Geometry check sheet. Reference: the model listing, model coordinates, mm. Face numbers are marked on the shaded views. A direction names the side the tool comes from. Round coordinates to 2 decimals unless told otherwise and drop trailing zeros. Loops run counter-clockwise (first coordinate to the right, second up) from the corner with the lowest first, then second, coordinate; pieces in that order, holes last.
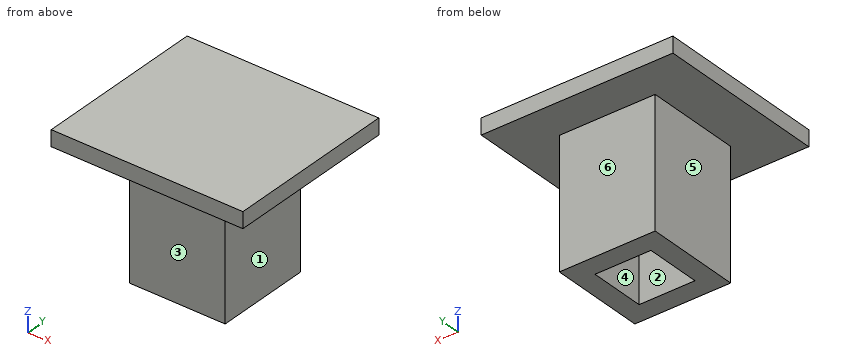
```python
from build123d import *

# Parameters (mm, degrees)
F0_W     = 152.4
F0_H     = 12.7
F1_DEPTH = 137.16
F2_W     = 76.2
F2_H     = 76.2
F3_DEPTH = 101.6
F4_W     = 44.45
F4_H     = 44.45
F5_DEPTH = 101.6


with BuildPart() as f1:
    # F0 (on Front) → F1 (new body)
    with BuildSketch(Plane.XZ):
        with Locations((76.2, 6.35)):
            Rectangle(F0_W, F0_H)
    extrude(amount=F1_DEPTH)

    # F2 (on face) → F3 (join)
    with BuildSketch(Plane(origin=(0, 0, 0), x_dir=(1, 0, 0), z_dir=(0, 0, -1))):
        with Locations((76.2, 68.58)):
            Rectangle(F2_W, F2_H)
    extrude(amount=F3_DEPTH)

    # F4 (on face) → F5 (cut)
    with BuildSketch(Plane(origin=(0, 0, -101.6), x_dir=(1, 0, 0), z_dir=(0, 0, -1))):
        with Locations((76.2, 68.58)):
            Rectangle(F4_W, F4_H)
    extrude(amount=-F5_DEPTH, mode=Mode.SUBTRACT)


solid = f1.part
```
1) Mould release check, pull along X, two halves, no side actions. Record for the marked faces 1, 2 and 3: +X half, -X half, draft (parallel to the pull), parting line (faces both ways), or undercut.
Report:
face 1: +X half
face 2: undercut
face 3: draft
2) Sectioned sample at C-C, the plane x = 50.5. Record the cut outline in (y, z), then the cut area to 3 significant figures.
Report:
outline: (-137.16, 0) - (-106.68, 0) - (-106.68, -101.6) - (-30.48, -101.6) - (-30.48, 0) - (0, 0) - (0, 12.7) - (-137.16, 12.7) - close
area: 9,480 mm2
3) Access from +Z, -Z, +X, -X, +Y, -Y to the whole of each face (thin tool, end or side, straight path). Record for the marked faces 4, 5 and 6.
Report:
face 4: -Z
face 5: -Z, -X, +Y, -Y
face 6: -Z, +X, -X, +Y
4) Sectioned sample at B-B, the plane y = -66.5. Record the cut outline in (x, z) (3 decimals).
Report:
outline: (0, 0) - (38.1, 0) - (38.1, -101.6) - (53.975, -101.6) - (53.975, 0) - (98.425, 0) - (98.425, -101.6) - (114.3, -101.6) - (114.3, 0) - (152.4, 0) - (152.4, 12.7) - (0, 12.7) - close
5) Gauge pin test, flat ends, axial feed: pin 1 (13.5 mm diameter, centred on x = 82, y = -60, fed in from -Z); pin 2 (13.5 mm diameter, centred on x = 72.5, z = -46, fed in from +Y); pin 3 (22 mm diameter, centred on y = -71, z = -70.5, fed in from -X). Record the tip position at first contact, or that the pin passes through.
Report:
pin 1: stops at z = 0
pin 2: stops at y = -30.48
pin 3: stops at x = 38.1
6) Sectioned sample at D-D, the plane y = -42. Record the cut outline in (x, z), then the cut area to 3 significant figures.
Report:
outline: (0, 0) - (38.1, 0) - (38.1, -101.6) - (114.3, -101.6) - (114.3, 0) - (152.4, 0) - (152.4, 12.7) - (0, 12.7) - close
area: 9,680 mm2
7) Sectioned sample at A-A, the plane z = -71. Record the cut outline in (x, y) (3 decimals), then the cut area to 3 significant figures.
Report:
outline: (38.1, -106.68) - (114.3, -106.68) - (114.3, -30.48) - (38.1, -30.48) - close; hole (53.975, -90.805) - (98.425, -90.805) - (98.425, -46.355) - (53.975, -46.355) - close
area: 3,830 mm2
8) Scan lines: line 1 along X through (y, z) = (-83, -47.5) (3 decimals); line 2 along Y through (x, z) = (73, -25) (3 decimals); line 3 along Z through (x, y) = (92, -10.5). Record each from-to range of solid material in increasing order.
Report:
line 1: x = 38.1 to 53.975, 98.425 to 114.3
line 2: y = -106.68 to -90.805, -46.355 to -30.48
line 3: z = 0 to 12.7
